CAD build for the part. Positions are in the model's coordinates, mm. Round coordinates to 2 decimals unless told otherwise and drop trailing zeros. Order: outer loops, then holes, each group sorted by start corner. A loop starts at its lowest first (then second) coordinate and runs counter-clockwise, first axis right, second up. Notation, with made-up numbers: M -20.5,89 L 2.5,89 A37 ccw 2.5,128 Z; hole C 63,-19.75 d11. An arc over 180 degrees is marked long. Answer as a JSON object with one key per item and string values.
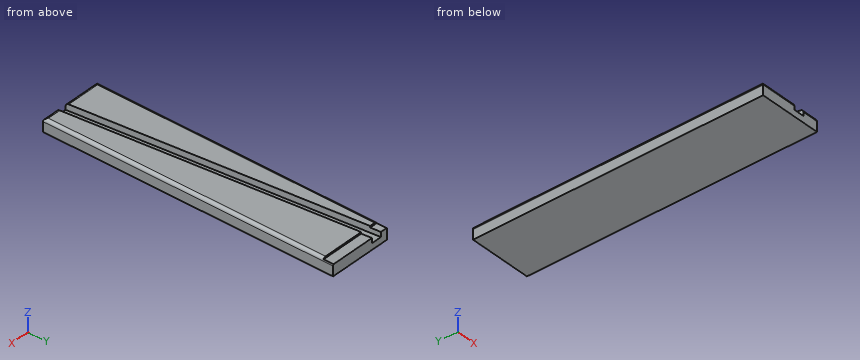
```python
from build123d import *

# Parameters (mm, degrees)
F1_DEPTH = 12.7
F2_DEPTH = 6.35
F3_START = 1.5
F3_DEPTH = 11.2
F4_START = 1.5
F4_DEPTH = 11.2
F5_R     = 3
F6_ANGLE = 180


with BuildPart() as f1:
    # F0 (on Top) → F1 (new body)
    with BuildSketch(Plane.XY):
        Polygon((-29.410376087, 163.8882011175), (-74.2387966365, 163.8882011175), (-74.2387966365, -118.2211643489), (-58.1500269473, -118.2211643489), align=None)
        Polygon((-17.8977344185, 173.8788356511), (-28.3925887197, 173.8788356511), (-29.410376087, 163.8882011175), (-58.1500269473, -118.2211643489), (-47.655172646, -118.2211643489), (-18.9155217858, 163.8882011175), align=None)
        Polygon((-10.7387966365, 163.8882011175), (-18.9155217858, 163.8882011175), (-47.655172646, -118.2211643489), (-42.4887966365, -118.2211643489), (-10.7387966365, -118.2211643489), align=None)
    extrude(amount=F1_DEPTH)

    # F0 (on Top) → F2 (cut)
    with BuildSketch(Plane.XY):
        Polygon((-17.8977344185, 173.8788356511), (-28.3925887197, 173.8788356511), (-29.410376087, 163.8882011175), (-58.1500269473, -118.2211643489), (-47.655172646, -118.2211643489), (-18.9155217858, 163.8882011175), align=None)
    extrude(amount=F2_DEPTH, mode=Mode.SUBTRACT)

    # F0 (on Top) → F3 (join)
    with BuildSketch(Plane.XY.offset(F3_START)):
        Polygon((-28.3925887197, 173.8788356511), (-74.2387966365, 173.8788356511), (-74.2387966365, 163.8882011175), (-29.410376087, 163.8882011175), align=None)
    extrude(amount=F3_DEPTH)

    # F0 (on Top) → F4 (join)
    with BuildSketch(Plane.XY.offset(F4_START)):
        Polygon((-10.7387966365, 173.8788356511), (-17.8977344185, 173.8788356511), (-18.9155217858, 163.8882011175), (-10.7387966365, 163.8882011175), align=None)
    extrude(amount=F4_DEPTH)

    # F5
    f5_edges = [f1.edges().sort_by_distance(p)[0] for p in [
        (-74.238797, 22.833518, 0),
        (-10.738797, 22.833518, 0),
        (-29.196985, -118.221164, 0),
        (-66.194412, -118.221164, 0),
    ]]
    fillet(f5_edges, radius=F5_R)


with BuildPart() as f1_1:
    # F6: moved
    add(f1.part.rotate(Axis((-13.7387966365, 24.3335183843, 0), (0, -1, 0)), F6_ANGLE))


solid = f1_1.part
```
Item 1: Saw through at B-B on y = -85. List the corners of the cut face in (x, z), and give its area (3 significant figures).
Worked answers:
{"outline": "M -16.74,-12.7 L 46.76,-12.7 L 46.76,-3 A3 ccw 43.76,0 L 27.29,0 L 27.29,-6.35 L 16.79,-6.35 L 16.79,0 L -13.74,0 A3 ccw -16.74,-3 Z", "area": "736 mm2"}
Item 2: Wall check: line 1 along Z through (x, y) = (16.5, -25); line 2 along X through (y, z) = (65, -1); line 3 along X through (y, z) = (-102, -1.5). Give the ranges that are in metal, low to high. Write a range as [from, to].
Worked answers:
{"line 1": "z = [-12.7, -6.35]", "line 2": "x = [-15.97, 1.51], [12.01, 46]", "line 3": "x = [-16.34, 18.53], [29.02, 46.36]"}
Item 3: Drop flat-ended pins along their axis: pin 1 Ø0.8 at (x, z) = (24, -1) entering from +Y; pin 2 Ø1 at (y, z) = (105.5, -2) entering from +X; pin 3 Ø3 at (x, y) = (33.5, 169) entering from +Z. Give the stop position or say it passes through.
Worked answers:
{"pin 1": "stops at y = 163.89", "pin 2": "stops at x = 46.72", "pin 3": "stops at z = -1.5"}
Item 4: Saw through at A-A on x = 24. List the corners of the cut face in (y, z).
Worked answers:
{"outline": "M -118.22,-12.7 L 173.88,-12.7 L 173.88,-1.5 L 163.89,-1.5 L 163.89,0 L -52.72,0 L -52.72,-6.35 L -118.22,-6.35 Z"}
